The model under review builds one solid part; all positions refer to its coordinate system, in mm. A direction names the side the tool comes from. Coordinates: 2 decimals unless noted, no trailing zeros. Write each loop counter-clockwise with the first axis right and the second up, starting at its lowest first coordinate (ties: lowest second). Pieces come first, ordered by that corner, then holes.
1) Add section A-A, the plane z = 59. State the section outline as (x, y) points.
2) For P1, Ø9.5, axis at y = 40.5, z = 48.5, coming from the +X side; P2, Ø1.5, axis at y = -16.5, z = 36.5, coming from the -X side; P3, Ø12, axis at y = -20, z = 61.5, coming from the -X side, all flat-tipped, find the tip position at first contact; note any pin that passes through.
3) Machinability: for faces 1 (the flat face through (-1, -10, 0)), 2 (the flat face through (-0.85, 34, 38)), which of the approach directions +Z, -Z, +X, -X, +Y, -Y give a long, thin tool a straight path to every point of the face, cutting with its end or side? Answer none if there is none.
4) For line 1 (Y direction, x = 0, z = 52); line 2 (X direction, y = 26.5, z = 51.5); line 3 (X direction, y = 19, z = 63), list the stretches that pass through material, from the lowest coordinate up.
5) Mouldability with a two-part tool opening along Y and no side actions: class faces 3 (the flat face through (0.85, 34, 38)), 4 (the cylindrical face through (-0.867, -3.905, 36.975)) as released by +Y, released by -Y, zero draft, split by the parting line, or undercut.
from build123d import *

# Parameters (mm, degrees)
SKETCH_R     = 50
SKETCH_R_2   = 4
PAD_DEPTH    = 75
FILLET_R     = 3
SKETCH001_R  = 3
SKETCH001_W  = 1.7
SKETCH001_H  = 50
POCKET_DEPTH = 75.001


with BuildPart() as part:
    # Sketch → Pad (new body)
    with BuildSketch(Plane.XY):
        Circle(SKETCH_R)
        Circle(SKETCH_R_2, mode=Mode.SUBTRACT)
    extrude(amount=PAD_DEPTH)

    # Fillet
    fillet_edges = [part.edges().sort_by_distance(p)[0] for p in [
        (-50, 0, 0),
        (-50, 0, 75),
    ]]
    fillet(fillet_edges, radius=FILLET_R)

    # Sketch001 (on Face5 of Fillet) → Pocket (cut, through all)
    with BuildSketch(Plane.XY.offset(75)):
        with Locations((0, 15)):
            Circle(SKETCH001_R)
        with Locations((0, 40)):
            Rectangle(SKETCH001_W, SKETCH001_H)
    extrude(amount=-POCKET_DEPTH, mode=Mode.SUBTRACT)


solid = part.part
Geometry results:
1. outline: (-0.85, 17.88) - (-0.85, 49.99) arc R50 ccw (long way) to (0.85, 49.99) - (0.85, 17.88) arc R3 cw (long way) to start; hole circle Ø8 at (0, 0)
2. P1: stops at x = 34.96
2. P2: stops at x = -47.45
2. P3: stops at x = -48
3. face 1: -Z, +X, -X, +Y, -Y
3. face 2: +Z, -Z, +Y
4. line 1: y = -50 to -4, 4 to 12
4. line 2: x = -42.4 to -0.85, 0.85 to 42.4
4. line 3: x = -46.25 to -0.85, 0.85 to 46.25
5. face 3: zero draft
5. face 4: undercut
